Autodesk Inventor part; units mm, degrees
ref_plane "YZ Plane" through (0, 0, 0) normal (1, 0, 0) x (0, 1, 0)
ref_plane "XZ Plane" through (0, 0, 0) normal (0, 1, 0) x (-1, 0, 0)
ref_plane "XY Plane" through (0, 0, 0) normal (0, 0, 1) x (1, 0, 0)
sketch "Sketch1" plane through (0, 0, 0) normal (0, 1, 0) x (-1, 0, 0)
  line L0 (0, 0) -> (-47, 0)
  line L1 (-47, 0) -> (-47, -43)
  line L2 (-47, -43) -> (0, -43)
  line L3 (0, -43) -> (0, 0)
  dimension "d0" = 43
  dimension "d1" = 47
extrude "Extrusion1" add sketch "Sketch1" along normal blind 3
sketch "Sketch2" plane through (0, 3, 0) normal (0, 1, 0) x (1, 0, 0)
  line L0 (47, 43) -> (0, 43)
  line L1 (0, 43) -> (0, 0)
  line L2 (6.5, 36.5) -> (40.5, 36.5) construction
  line L3 (40.5, 36.5) -> (40.5, 6.5) construction
  line L4 (40.5, 6.5) -> (6.5, 6.5) construction
  line L5 (6.5, 6.5) -> (6.5, 36.5) construction
  point P0 (23.5, 36.5)
  point P1 (23.5, 43)
  point P2 (6.5, 21.5)
  point P3 (0, 21.5)
  dimension "d4" = 6.5
  dimension "d5" = 6.5
hole "Hole1" at (6.5, 3, -6.5) at (6.5, 3, -36.5) at (40.5, 3, -36.5) at (40.5, 3, -6.5) direction (0, -1, 0) diameter 4 end through all countersink diameter 8.5 countersink angle 90
sketch "Sketch3" plane through (0, 0, 0) normal (0, -1, 0) x (1, 0, 0)
  line L0 (0, 0) -> (47, 0)
  line L1 (21.4, 0) -> (25.6, 0)
  line L2 (25.6, 0) -> (25.6, -3)
  line L3 (25.6, -3) -> (21.4, -3)
  line L4 (21.4, -3) -> (21.4, 0)
  point P0 (23.5, -3)
  point P1 (23.5, 0)
  dimension "d13" = 4.2
  dimension "d14" = 3
extrude "Extrusion2" add sketch "Sketch3" along normal blind 6.2
sketch "Sketch4" plane through (0, 3, 0) normal (0, 1, 0) x (1, 0, 0)
  line L0 (47, 43) -> (0, 43)
  line L1 (0, 43) -> (0, 0)
  circle A0 centre (23.5, 21.5) radius 1.5
  circle A1 centre (23.5, 26.5) radius 1.5
  circle A2 centre (18.7447, 23.0451) radius 1.5
  circle A3 centre (20.5611, 17.4549) radius 1.5
  circle A4 centre (26.4389, 17.4549) radius 1.5
  circle A5 centre (28.2553, 23.0451) radius 1.5
  circle A6 centre (23.5, 11.5) radius 1.5
  circle A7 centre (29.9279, 13.8396) radius 1.5
  circle A8 centre (33.3481, 19.7635) radius 1.5
  circle A9 centre (32.1603, 26.5) radius 1.5
  circle A10 centre (26.9202, 30.8969) radius 1.5
  circle A11 centre (20.0798, 30.8969) radius 1.5
  circle A12 centre (14.8397, 26.5) radius 1.5
  circle A13 centre (13.6519, 19.7635) radius 1.5
  circle A14 centre (17.0721, 13.8396) radius 1.5
  point P0 (23.5, 43)
  point P1 (0, 21.5)
  dimension "d17" = 3
  dimension "d18" = 3
  dimension "d19" = 5
  dimension "d22" = 360
  dimension "d24" = 3
  dimension "d25" = 10
  dimension "d28" = 360
extrude "Extrusion3" cut sketch "Sketch4" against normal through all
fillet "Fillet1" radius 6 4 edges at (0, 1.5, -43) (0, 1.5, 0) (47, 1.5, 0) (47, 1.5, -43)
equation "\"d5\" = d4"
equation "\"d18\" = d17"
equation "\"d24\" = d17"
properties part number "dht22_case_top"
Source: CAD feature listing. Evaluate the final solid. Frame: model axes, mm. Give positions to 0.01 mm unless a question says otherwise; leave off trailing zeros. Write each loop counter-clockwise with the first axis right and the second up, starting at its lowest first coordinate (ties: lowest second). Pieces come first, ordered by that corner, then holes. Notation, with made-up numbers: M 64,80 L 83,80 A12 ccw 83,101 Z; hole C 35,-27 d7. An arc over 180 degrees is marked long. Return JSON: item names as keys, results as strings. Group by question number.
1) Cut plane D-D, the plane y = -2.25. Output: boundary loops of the cut face in (x, z), plus the area to 3 significant figures.
2) Pull-direction query (X, two-part tool) for faces 1 (the face through (23, -6.2, -1)), 2 (the face through (21.4, -3, -2)), 3 (the face through (31.965, 1.521, -27.987)); classes: pulls with the +X half, pulls with the -X half, needs draft (parallel to the pull), parting line crosses it, or undercut.
3) Cut plane C-C, the plane x = 7.5. Give the number of separate pieces and of enclosed holes in the cut face, plus the area to 3 significant figures.
4) Cut plane A-A, the plane z = -26.5. Output: boundary loops of the cut face in (x, y).
5) Material intervals for line 1 along X through (y, z) = (0.65, -36.5); line 2 along X through (y, z) = (1.25, -35.5); line 3 along Z through (x, y) = (6.5, 0.4), sorted ascending. Write a range as [from, to].
6) Cut plane B-B, the plane x = 23.5. Output: boundary loops of the cut face in (y, z), plus the area to 3 significant figures.
7) Pin query (flat end, axial travel): P1, Ø8, axis at x = 10.5, z = -7.5, coming from the -Y side; P2, Ø2.5, axis at y = -3, z = -1.5, coming from the -X side; P3, Ø2.5, axis at x = 14.84, z = -26.5, coming from the -Y side; P4, Ø5, axis at x = 40.5, z = -6.5, coming from the +Y side. Return the tip coordinate at first contact, or that it passes through.
Recorded:
{
 "1": {"outline": "M 21.4,-3 L 25.6,-3 L 25.6,0 L 21.4,0 Z", "area": "12.6 mm²"},
 "2": {"face 1": "needs draft", "face 2": "pulls with the -X half", "face 3": "undercut"},
 "3": {"separate pieces": "3", "enclosed holes": "0", "area": "97.2 mm²"},
 "4": {"outline": "M 0,0 L 13.34,0 L 13.34,3 L 0,3 Z; M 16.34,0 L 22,0 L 22,3 L 16.34,3 Z; M 25,0 L 30.66,0 L 30.66,3 L 25,3 Z; M 33.66,0 L 47,0 L 47,3 L 33.66,3 Z"},
 "5": {"line 1": "x = [0, 4.5], [8.5, 38.5], [42.5, 47]", "line 2": "x = [0, 4.21], [8.79, 38.21], [42.79, 47]", "line 3": "z = [-43, -38.5], [-34.5, -8.5], [-4.5, 0]"},
 "6": {"outline": "M -6.2,-3 L 0,-3 L 0,-10 L 3,-10 L 3,0 L -6.2,0 Z; M 0,-43 L 3,-43 L 3,-28 L 0,-28 Z; M 0,-25 L 3,-25 L 3,-23 L 0,-23 Z; M 0,-20 L 3,-20 L 3,-13 L 0,-13 Z", "area": "121 mm²"},
 "7": {"P1": "stops at y = 0", "P2": "stops at x = 21.4", "P3": "passes through", "P4": "stops at y = 1.25"}
}
